from build123d import *

# Parameters (mm, degrees)
SKETCH1_W           = 20
SKETCH1_H           = 100
BOSS_EXTRUDE1_DEPTH = 20
SKETCH2_W           = 10
SKETCH2_H           = 40
CUT_EXTRUDE1_DEPTH  = 55.772255751
SKETCH3_R           = 2
CUT_EXTRUDE2_DEPTH  = 58.445626465
FILLET1_R           = 10
SKETCH4_W           = 20
SKETCH4_H           = 15
BOSS_EXTRUDE2_DEPTH = 20
SKETCH5_R           = 2
CUT_EXTRUDE3_DEPTH  = 68.082039325
CUT_EXTRUDE4_REACH  = 110.167
SKETCH6_W           = 10
SKETCH6_H           = 20
FILLET2_R           = 7.5


with BuildPart() as part:
    # Sketch1 → Boss-Extrude1 (new body)
    with BuildSketch(Plane(origin=(0, 0, 0), x_dir=(1, 0, 0), z_dir=(0, 1, 0))):
        Rectangle(SKETCH1_W, SKETCH1_H)
    extrude(amount=BOSS_EXTRUDE1_DEPTH)

    # Sketch2 → Cut-Extrude1 (cut, through all)
    with BuildSketch(Plane(origin=(0, 20, 0), x_dir=(1, 0, 0), z_dir=(0, 1, 0))):
        with Locations((0, -30)):
            Rectangle(SKETCH2_W, SKETCH2_H)
    extrude(amount=-CUT_EXTRUDE1_DEPTH, mode=Mode.SUBTRACT)

    # Sketch3 → Cut-Extrude2 (cut, through all)
    with BuildSketch(Plane(origin=(10, 0, 0), x_dir=(0, 0, -1), z_dir=(1, 0, 0))):
        with Locations((-40, 10)):
            Circle(SKETCH3_R)
        with Locations((-20, 10)):
            Circle(SKETCH3_R)
    extrude(amount=-CUT_EXTRUDE2_DEPTH, mode=Mode.SUBTRACT)

    # Fillet1
    fillet1_edges = [part.edges().sort_by_distance(p)[0] for p in [
        (7.5, 0, 50),
        (-7.5, 0, 50),
        (-7.5, 20, 50),
        (7.5, 20, 50),
    ]]
    fillet(fillet1_edges, radius=FILLET1_R - 0.0001)  # a hair under: the kernel refuses the full size

    # Sketch4 → Boss-Extrude2 (add)
    with BuildSketch(Plane(origin=(0, 20, 0), x_dir=(1, 0, 0), z_dir=(0, 1, 0))):
        with Locations((0, 42.5)):
            Rectangle(SKETCH4_W, SKETCH4_H)
    boss_extrude2 = extrude(amount=BOSS_EXTRUDE2_DEPTH)

    # Mirror1: Boss-Extrude2 across plane
    add(boss_extrude2.mirror(Plane.ZX.offset(10)))

    # Sketch5 → Cut-Extrude3 (cut, through all)
    with BuildSketch(Plane.ZY.offset(10)):
        with Locations((-42.5, 35)):
            Circle(SKETCH5_R)
        with Locations((-42.5, -15)):
            Circle(SKETCH5_R)
    extrude(amount=-CUT_EXTRUDE3_DEPTH, mode=Mode.SUBTRACT)

    # Sketch6 → Cut-Extrude4 (cut, up to next)
    with BuildSketch(Plane(origin=(0, 0, -50), x_dir=(-1, 0, 0), z_dir=(0, 0, -1)), mode=Mode.PRIVATE) as cut_extrude4_sk1:
        with Locations((0, 30)):
            Rectangle(SKETCH6_W, SKETCH6_H)
    cut_extrude4_tool1 = extrude(cut_extrude4_sk1.sketch, amount=-CUT_EXTRUDE4_REACH, mode=Mode.PRIVATE) & part.part
    # Sketch6 → Cut-Extrude4 (cut, up to next)
    with BuildSketch(Plane(origin=(0, 0, -50), x_dir=(-1, 0, 0), z_dir=(0, 0, -1)), mode=Mode.PRIVATE) as cut_extrude4_sk2:
        with Locations((0, -10)):
            Rectangle(SKETCH6_W, SKETCH6_H)
    cut_extrude4_tool2 = extrude(cut_extrude4_sk2.sketch, amount=-CUT_EXTRUDE4_REACH, mode=Mode.PRIVATE) & part.part
    add(cut_extrude4_tool1.solids().sort_by_distance((0, 30, -50))[0], mode=Mode.SUBTRACT)
    add(cut_extrude4_tool2.solids().sort_by_distance((0, -10, -50))[0], mode=Mode.SUBTRACT)

    # Fillet2
    fillet2_edges = [part.edges().sort_by_distance(p)[0] for p in [
        (-7.5, 40, -35),
        (-7.5, 40, -50),
        (7.5, 40, -35),
        (7.5, 40, -50),
        (7.5, -20, -35),
        (7.5, -20, -50),
        (-7.5, -20, -35),
        (-7.5, -20, -50),
    ]]
    fillet(fillet2_edges, radius=FILLET2_R - 0.0001)  # a hair under: the kernel refuses the full size


solid = part.part
The model under review builds one solid part; all positions refer to its coordinate system, in mm. A direction names the side the tool comes from. Round coordinates to 2 decimals unless told otherwise and drop trailing zeros. Loops run counter-clockwise (first coordinate to the right, second up) from the corner with the lowest first, then second, coordinate; pieces in that order, holes last. Notation, with made-up numbers: (-13.75, 38.25) -> (32.25, 38.25) arc R21 cw to (32.25, 50.25) -> close; hole circle Ø7 at (-23.75, 85.25). An arc over 180 degrees is marked (long way). Write item = value, one per line. Start each with the question number.
Item 1: Mouldability with a two-part tool opening along X and no side actions: class faces 6 (the flat face through (5, 30, -43)), 7 (the flat face through (-5, 10, 30)), 8 (the flat face through (0, 10, -50)), 9 (the flat face through (10, 10, -10)) as released by +X, released by -X, zero draft, split by the parting line, or undercut.
Item 2: Insertion check: pin 1 (5.5 mm diameter, centred on x = 7, y = -7, fed in from +Z); pin 2 (6 mm diameter, centred on x = 1.5, z = -7, fed in from +Y); pin 3 (1.5 mm diameter, centred on x = -6.5, z = -13, fed in from -Y). Each pin has a flat end and moves straight along its axis. Give the tip position at first contact, or say it passes through.
Item 3: Take a section at B-B on y = 24. Give the boundary of the cut face in (x, z).
Item 4: Take a section at D-D on x = 1.25. Give the boundary of the cut face in (y, z), plus the area to 3 significant figures.
Item 5: Take a section at C-C on y = 34. Give the boundary of the cut face in (x, z), plus the area to 3 significant figures.
Item 6: For faces 1 (the flat face through (5, 10, 30)), 2 (the flat face through (-5, 30, -43)), 3 (the flat face through (7, -6, -35)), 4 (the flat face through (-5, -10, -43)), 5 (the cylindrical face through (-7.535, 33.048, -42.934)), list the 3-axis set-ups (+Z, -Z, +X, -X, +Y, -Y) from which the entire face can be reached by the end or side of a thin tool; tool diameter is ignored.
Item 7: To check wall thickness, follow L1, parallel to Y at x = 6.8, z = -42.5; L2, parallel to X at y = -3, z = -40.5; L3, parallel to Y at x = -6.4, z = 20. State the ranges of each line that lie inside material, in increasing order.
Item 8: Take a section at A-A on z = 33. Give the boundary of the cut face in (x, y), plus the area to 3 significant figures.
Result:
q1.face_6 = undercut
q1.face_7 = undercut
q1.face_8 = zero draft
q1.face_9 = released by +X
q2.pin_1 = -35
q2.pin_2 = 20
q2.pin_3 = 0
q3.outline = (-10, -50) -> (-5, -50) -> (-5, -35) -> (-10, -35) -> close; (5, -50) -> (10, -50) -> (10, -35) -> (5, -35) -> close
q4.outline = (0, -50) -> (20, -50) -> (20, 10) -> (0, 10) -> close
q4.area = 1,200 mm²
q5.outline = (-10, -49.85) -> (-5, -49.85) -> (-5, -44.23) -> (-10, -44.23) -> close; (-10, -40.77) -> (-5, -40.77) -> (-5, -35.15) -> (-10, -35.15) -> close; (5, -49.85) -> (10, -49.85) -> (10, -44.23) -> (5, -44.23) -> close; (5, -40.77) -> (10, -40.77) -> (10, -35.15) -> (5, -35.15) -> close
q5.area = 112 mm²
q6.face_1 = +Z, +Y, -Y
q6.face_2 = +Z, -Z, +Y
q6.face_3 = +Z, +X, -X, -Y
q6.face_4 = +Z, -Z, -Y
q6.face_5 = +X, -X
q7.L1 = -20 to -17, -13 to 33, 37 to 40
q7.L2 = -10 to -5, 5 to 10
q7.L3 = 0 to 8, 12 to 20
q8.outline = (-10, 0) -> (-5, 0) -> (-5, 20) -> (-10, 20) -> close; (5, 0) -> (10, 0) -> (10, 20) -> (5, 20) -> close
q8.area = 200 mm²
